Solid Edge part; units mm, degrees
sketch "Sketch1" plane through (0, 0, 0) normal (0, 0, 1) x (1, 0, 0)
  line L0 (-1.25, -25.5) -> (1.25, -25.5)
  line L1 (1.25, -25.5) -> (1.25, 25.5)
  line L2 (1.25, 25.5) -> (-1.25, 25.5)
  line L3 (-1.25, 25.5) -> (-1.25, -25.5)
  dimension "D1" = 1.25
  dimension "D2" = 1.25
extrude "Protrusion1" add sketch "Sketch1" along normal blind 2.7
sketch "Sketch2" plane through (0, 0, 2.7) normal (0, 0, 1) x (0, 1, 0)
  line L0 (-25.1, -0.325) -> (25.1, -0.325)
  line L1 (25.1, -0.325) -> (25.1, 0.325)
  line L2 (25.1, 0.325) -> (-25.1, 0.325)
  line L3 (-25.1, 0.325) -> (-25.1, -0.325)
  dimension "D1" = 25.1
  dimension "D2" = 25.1
extrude "Extrusionsausprägung_2" add sketch "Sketch2" along normal blind 6
sketch "Sketch3" plane through (0.325, 0, 5.7) normal (1, 0, 0) x (0, 1, 0)
  line L0 (-21.79, 3) -> (-19.89, 3)
  line L1 (-19.89, 3) -> (-19.89, -3)
  line L2 (-19.89, -3) -> (-21.79, -3)
  line L3 (-21.79, -3) -> (-21.79, 3)
  line L4 (-19.185, 3) -> (-17.285, 3)
  line L5 (-17.285, 3) -> (-17.285, -3)
  line L6 (-17.285, -3) -> (-19.185, -3)
  line L7 (-19.185, -3) -> (-19.185, 3)
  line L8 (-16.58, 3) -> (-14.68, 3)
  line L9 (-14.68, 3) -> (-14.68, -3)
  line L10 (-14.68, -3) -> (-16.58, -3)
  line L11 (-16.58, -3) -> (-16.58, 3)
  line L12 (-13.975, 3) -> (-12.075, 3)
  line L13 (-12.075, 3) -> (-12.075, -3)
  line L14 (-12.075, -3) -> (-13.975, -3)
  line L15 (-13.975, -3) -> (-13.975, 3)
  line L16 (-11.37, 3) -> (-9.47, 3)
  line L17 (-9.47, 3) -> (-9.47, -3)
  line L18 (-9.47, -3) -> (-11.37, -3)
  line L19 (-11.37, -3) -> (-11.37, 3)
  line L20 (-8.765, 3) -> (-6.865, 3)
  line L21 (-6.865, 3) -> (-6.865, -3)
  line L22 (-6.865, -3) -> (-8.765, -3)
  line L23 (-8.765, -3) -> (-8.765, 3)
  line L24 (-6.16, 3) -> (-4.26, 3)
  line L25 (-4.26, 3) -> (-4.26, -3)
  line L26 (-4.26, -3) -> (-6.16, -3)
  line L27 (-6.16, -3) -> (-6.16, 3)
  line L28 (-3.555, 3) -> (-1.655, 3)
  line L29 (-1.655, 3) -> (-1.655, -3)
  line L30 (-1.655, -3) -> (-3.555, -3)
  line L31 (-3.555, -3) -> (-3.555, 3)
  line L32 (-0.95, 3) -> (0.95, 3)
  line L33 (0.95, 3) -> (0.95, -3)
  line L34 (0.95, -3) -> (-0.95, -3)
  line L35 (-0.95, -3) -> (-0.95, 3)
  line L36 (-24.395, 3) -> (-22.495, 3)
  line L37 (-22.495, 3) -> (-22.495, -3)
  line L38 (-22.495, -3) -> (-24.395, -3)
  line L39 (-24.395, -3) -> (-24.395, 3)
  dimension "D1" = 24.395
extrude "Cutout1" cut sketch "Sketch3" against normal through all
mirror "Mirror1" about plane through (0, 0, 0) normal (0, -1, 0) of "Cutout1"
Could you check a few things on this model? Use its own coordinates, in mm. Give positions to 0.01 mm unless a question says otherwise; leave off trailing zeros. Loops run counter-clockwise (first coordinate to the right, second up) from the corner with the lowest first, then second, coordinate; pieces in that order, holes last. Notation, with made-up numbers: M 68,-37.5 L 72,-37.5 A33 ccw 72,1.5 Z; hole C 49,-3.75 d1. An arc over 180 degrees is marked long. Answer as a JSON object with one key per item and string values.
Q1. If we mould it in two halves opening along Y, with no side actions, what happens to faces 1 (the flat face through (0, 0, 2.7)), 2 (the flat face through (-1.25, 0, 1)), 3 (the flat face through (0, -25.5, 1))? For each: pulls with the +Y half, pulls with the -Y half, needs draft (parallel to the pull), parting line crosses it, or undercut.
Values found:
{"face 1": "undercut", "face 2": "needs draft", "face 3": "pulls with the -Y half"}
Q2. If I drill on probe 1 along Z at (x, y) = (-0.8, -8); probe 2 along X at (y, z) = (1, 6) (3 decimals), over which ranges is the centre line in solid material (lowest first)? Write a range as [from, to].
Values found:
{"probe 1": "z = [0, 2.7]", "probe 2": "x = [-0.325, 0.325]"}
Q3. Suppose I cut it at B-B, the plane x = -0.75. List the corners of the cut face in (y, z) for me.
Values found:
{"outline": "M -25.5,0 L 25.5,0 L 25.5,2.7 L -25.5,2.7 Z"}
Q4. Suppose I cut it at A-A, the plane z = 4.75. State how many separate pieces and enclosed holes the cut face has, plus the area to 4 significant figures.
Values found:
{"separate pieces": "20", "enclosed holes": "0", "area": "9.165 mm²"}
Q5. Suppose I cut it at C-C, the plane y = 16. List the corners of the cut face in (x, z) for me.
Values found:
{"outline": "M -1.25,0 L 1.25,0 L 1.25,2.7 L -1.25,2.7 Z"}
Q6. For P1, Ø0.6, axis at y = -12, z = 6, coming from the +X side (3 decimals); P2, Ø0.6, axis at y = 12, z = 5.5, coming from the -X side (3 decimals); P3, Ø0.7, axis at x = 0, z = 5, coming from the +Y side, each with a flat end and sliding along its axis, tell me the tip position at first contact or that it passes through.
Values found:
{"P1": "stops at x = 0.325", "P2": "stops at x = -0.325", "P3": "stops at y = 25.1"}
